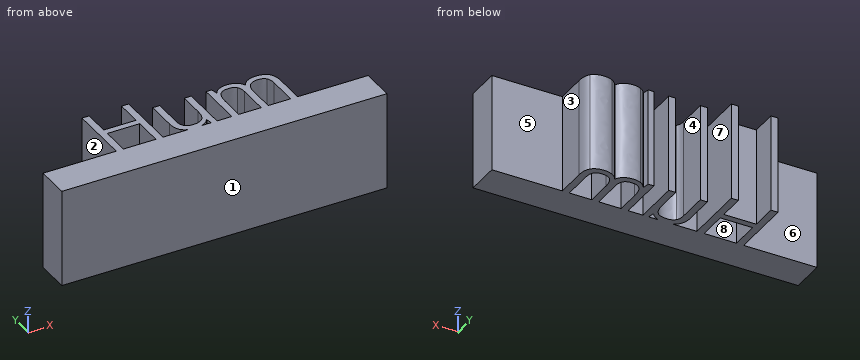
from build123d import *

# Parameters (mm, degrees)
F1_DEPTH = 15


with BuildPart() as f1:
    # F0 (on Top) → F1 (new body)
    with BuildSketch(Plane.XY):
        with BuildLine():
            Line((0, 5.1869419025), (0, 0))
            Line((0, 0), (50, 0))
            Line((50, 0), (50, 5.1869419025))
            Line((50, 5.1869419025), (39.1645775294, 5.1869419025))
            Line((39.1645775294, 5.1869419025), (38.091016748, 5.1869419025))
            Line((38.091016748, 5.1869419025), (34.6382131539, 5.1869419025))
            Line((34.6382131539, 5.1869419025), (33.5625798614, 5.1869419025))
            Line((33.5625798614, 5.1869419025), (30.1180663119, 5.1869419025))
            Line((30.1180663119, 5.1869419025), (29.0424330194, 5.1869419025))
            Line((29.0424330194, 5.1869419025), (26.7626707424, 5.1869419025))
            Line((26.7626707424, 5.1869419025), (25.8756359655, 5.1869419025))
            Line((25.8756359655, 5.1869419025), (24.3593894687, 5.1869419025))
            add(Edge.make_bspline(
                [(24.3593894687, 5.1869419025), (23.9221630132, 5.0563736994), (23.4072751728, 5.0563736994)],
                knots=[0.3156013684, 0.3156013684, 0.3156013684, 1, 1, 1], degree=2))
            add(Edge.make_bspline(
                [(23.4072751728, 5.0563736994), (22.8106948217, 5.0563736994), (22.3523760863, 5.1869419025)],
                knots=[0, 0, 0, 0.4605661865, 0.4605661865, 0.4605661865], degree=2))
            Line((22.3523760863, 5.1869419025), (18.4664085652, 5.1869419025))
            Line((18.4664085652, 5.1869419025), (17.3659051387, 5.1869419025))
            Line((17.3659051387, 5.1869419025), (12.3773707744, 5.1869419025))
            Line((12.3773707744, 5.1869419025), (11.2768673479, 5.1869419025))
            Line((11.2768673479, 5.1869419025), (0, 5.1869419025))
        make_face()
        Polygon((11.2768673479, 14.6562453968), (11.2768673479, 5.1869419025), (12.3773707744, 5.1869419025), (12.3773707744, 9.6428408985), (17.3659051387, 9.6428408985), (17.3659051387, 5.1869419025), (18.4664085652, 5.1869419025), (18.4664085652, 14.6562453968), (17.3659051387, 14.6562453968), (17.3659051387, 10.6272837), (12.3773707744, 10.6272837), (12.3773707744, 14.6562453968), align=None)
        with BuildLine():
            Line((38.091016748, 5.1869419025), (39.1645775294, 5.1869419025))
            Line((39.1645775294, 5.1869419025), (39.1645775294, 9.816931836))
            add(Edge.make_bspline(
                [(38.5656218039, 11.7972162503), (39.1645775294, 11.1785716688), (39.1645775294, 9.816931836)],
                knots=[0, 0, 0, 1, 1, 1], degree=2))
            add(Edge.make_bspline(
                [(36.7625370938, 12.4158608318), (37.9666660783, 12.4158608318), (38.5656218039, 11.7972162503)],
                knots=[0, 0, 0, 1, 1, 1], degree=2))
            add(Edge.make_bspline(
                [(35.3894984497, 12.0915128351), (35.991562942, 12.4158608318), (36.7625370938, 12.4158608318)],
                knots=[0, 0, 0, 1, 1, 1], degree=2))
            add(Edge.make_bspline(
                [(34.4703397499, 11.2096593362), (34.7874339575, 11.7671648385), (35.3894984497, 12.0915128351)],
                knots=[0, 0, 0, 1, 1, 1], degree=2))
            Line((34.4703397499, 11.2096593362), (34.4185269708, 11.2096593362))
            add(Edge.make_bspline(
                [(32.2423902519, 12.4158608318), (33.9066167141, 12.4158608318), (34.4185269708, 11.2096593362)],
                knots=[0, 0, 0, 1, 1, 1], degree=2))
            add(Edge.make_bspline(
                [(31.001992322, 12.1236367581), (31.5563890576, 12.4158608318), (32.2423902519, 12.4158608318)],
                knots=[0, 0, 0, 1, 1, 1], degree=2))
            add(Edge.make_bspline(
                [(30.1429364458, 11.3132848942), (30.4475955865, 11.8314126845), (31.001992322, 12.1236367581)],
                knots=[0, 0, 0, 1, 1, 1], degree=2))
            Line((30.1429364458, 11.3132848942), (30.0911236668, 11.3132848942))
            Line((30.0911236668, 11.3132848942), (29.9170327293, 12.2852926287))
            Line((29.9170327293, 12.2852926287), (29.0424330194, 12.2852926287))
            Line((29.0424330194, 12.2852926287), (29.0424330194, 5.1869419025))
            Line((29.0424330194, 5.1869419025), (30.1180663119, 5.1869419025))
            Line((30.1180663119, 5.1869419025), (30.1180663119, 8.9112444587))
            add(Edge.make_bspline(
                [(30.5874900899, 10.8967101509), (30.1180663119, 10.2915368919), (30.1180663119, 8.9112444587)],
                knots=[0, 0, 0, 1, 1, 1], degree=2))
            add(Edge.make_bspline(
                [(32.0662268032, 11.5018834099), (31.0569138678, 11.5018834099), (30.5874900899, 10.8967101509)],
                knots=[0, 0, 0, 1, 1, 1], degree=2))
            add(Edge.make_bspline(
                [(33.1998904082, 11.0780548775), (32.837200955, 11.5018834099), (32.0662268032, 11.5018834099)],
                knots=[0, 0, 0, 1, 1, 1], degree=2))
            add(Edge.make_bspline(
                [(33.5625798614, 9.8044967691), (33.5625798614, 10.654226345), (33.1998904082, 11.0780548775)],
                knots=[0, 0, 0, 1, 1, 1], degree=2))
            Line((33.5625798614, 9.8044967691), (33.5625798614, 5.1869419025))
            Line((33.5625798614, 5.1869419025), (34.6382131539, 5.1869419025))
            Line((34.6382131539, 5.1869419025), (34.6382131539, 9.1516557534))
            add(Edge.make_bspline(
                [(35.1179994877, 10.9257253071), (34.6382131539, 10.3495672044), (34.6382131539, 9.1516557534)],
                knots=[0, 0, 0, 1, 1, 1], degree=2))
            add(Edge.make_bspline(
                [(36.6008812233, 11.5018834099), (35.5977858214, 11.5018834099), (35.1179994877, 10.9257253071)],
                knots=[0, 0, 0, 1, 1, 1], degree=2))
            add(Edge.make_bspline(
                [(37.7283272948, 11.0780548775), (37.3656378417, 11.5018834099), (36.6008812233, 11.5018834099)],
                knots=[0, 0, 0, 1, 1, 1], degree=2))
            add(Edge.make_bspline(
                [(38.091016748, 9.8044967691), (38.091016748, 10.654226345), (37.7283272948, 11.0780548775)],
                knots=[0, 0, 0, 1, 1, 1], degree=2))
            Line((38.091016748, 9.8044967691), (38.091016748, 5.1869419025))
        make_face()
        with BuildLine():
            add(Edge.make_bspline(
                [(22.3523760863, 5.1869419025), (21.8155745788, 5.3398686822), (21.4684409818, 5.6719095142)],
                knots=[0.4605661865, 0.4605661865, 0.4605661865, 1, 1, 1], degree=2))
            Line((22.3523760863, 5.1869419025), (24.3593894687, 5.1869419025))
            add(Edge.make_bspline(
                [(24.7461173828, 5.3351264505), (24.5610106604, 5.2471517008), (24.3593894687, 5.1869419025)],
                knots=[0, 0, 0, 0.3156013684, 0.3156013684, 0.3156013684], degree=2))
            add(Edge.make_bspline(
                [(25.6621673159, 6.1382245254), (25.3326380413, 5.6138792017), (24.7461173828, 5.3351264505)],
                knots=[0, 0, 0, 1, 1, 1], degree=2))
            Line((25.6621673159, 6.1382245254), (25.7201976284, 6.1382245254))
            Line((25.7201976284, 6.1382245254), (25.8756359655, 5.1869419025))
            Line((25.8756359655, 5.1869419025), (26.7626707424, 5.1869419025))
            Line((26.7626707424, 5.1869419025), (26.7626707424, 12.2852926287))
            Line((26.7626707424, 12.2852926287), (25.6870374498, 12.2852926287))
            Line((25.6870374498, 12.2852926287), (25.6870374498, 8.554772539))
            add(Edge.make_bspline(
                [(25.1730546819, 6.5661980801), (25.6870374498, 7.1744801058), (25.6870374498, 8.554772539)],
                knots=[0, 0, 0, 1, 1, 1], degree=2))
            add(Edge.make_bspline(
                [(23.5440609094, 5.9579160544), (24.659071914, 5.9579160544), (25.1730546819, 6.5661980801)],
                knots=[0, 0, 0, 1, 1, 1], degree=2))
            add(Edge.make_bspline(
                [(22.307808002, 6.3848533535), (22.7026213781, 5.9579160544), (23.5440609094, 5.9579160544)],
                knots=[0, 0, 0, 1, 1, 1], degree=2))
            add(Edge.make_bspline(
                [(21.9129946258, 7.6801728291), (21.9129946258, 6.8117906527), (22.307808002, 6.3848533535)],
                knots=[0, 0, 0, 1, 1, 1], degree=2))
            Line((21.9129946258, 7.6801728291), (21.9129946258, 12.2852926287))
            Line((21.9129946258, 12.2852926287), (20.8249262663, 12.2852926287))
            Line((20.8249262663, 12.2852926287), (20.8249262663, 7.6407951171))
            add(Edge.make_bspline(
                [(21.4684409818, 5.6719095142), (20.8249262663, 6.287445329), (20.8249262663, 7.6407951171)],
                knots=[0, 0, 0, 1, 1, 1], degree=2))
        make_face()
        with BuildLine():
            Line((24.3593894687, 5.1869419025), (22.3523760863, 5.1869419025))
            add(Edge.make_bspline(
                [(23.4072751728, 5.0563736994), (22.8106948217, 5.0563736994), (22.3523760863, 5.1869419025)],
                knots=[0, 0, 0, 0.4605661865, 0.4605661865, 0.4605661865], degree=2))
            add(Edge.make_bspline(
                [(24.3593894687, 5.1869419025), (23.9221630132, 5.0563736994), (23.4072751728, 5.0563736994)],
                knots=[0.3156013684, 0.3156013684, 0.3156013684, 1, 1, 1], degree=2))
        make_face()
    extrude(amount=F1_DEPTH)


solid = f1.part
The listing builds one solid part. Answer for the finished solid, in the listing's coordinates (mm). Face numbers are marked on the shaded views. A direction names the side the tool comes from. Coordinates: 2 decimals unless noted, no trailing zeros. Loops run counter-clockwise (first coordinate to the right, second up) from the corner with the lowest first, then second, coordinate; pieces in that order, holes last. Notation, with made-up numbers: (54.25, 74) -> (107.25, 74) arc R16 ccw to (107.25, 95) -> close; hole circle Ø3 at (37.25, 71.5). An arc over 180 degrees is marked (long way). Write item = value, one per line. Start each with the question number.
1) A cutting plane is placed at A-A (y = 13.75). Give the vertices of the cut face in (x, z), then the cut area to 3 significant figures.
2) The mould has two halves that part along X. Classify the marked faces 1, 2, 3 and 4: released by +X, released by -X, zero draft, split by the parting line, or undercut.
3) Given pin 1 Ø3.5 at (y, z) = (7, 6.5) entering from -X; pin 2 Ø4 at (y, z) = (9.5, 10.5) entering from +X; pin 3 Ø0.9 at (x, z) = (26.5, 9.5) entering from +Y, each flat-ended and moving along its own axis, determine where each tip first touches the part or whether it passes through.
4) A cutting plane is placed at B-B (x = 15). Give the vertices of the cut face in (y, z).
5) Straight lines are drawn through the part: line 1 (X direction, y = 12.5, z = 11); line 2 (Y direction, x = 8, z = 5.5). For each, find the intervals that lie inside material, in ascending order. Write a range as from..to.
6) A cutting plane is placed at D-D (x = 44). Give the vertices of the cut face in (y, z).
7) A tool of negligible diameter and unlimited length cuts with its end or side. For the marked faces 5, 6, 7 and 8, from which of +Z, -Z, +X, -X, +Y, -Y can it reach the whole face along a straight path? Write none if from no direction.
8) A cutting plane is placed at C-C (z = 2.5). Count the separate pieces of the cut face and the enclosed holes in it, then the cut area to 3 significant figures.
Responses:
q1.outline = (11.28, 0) -> (12.38, 0) -> (12.38, 15) -> (11.28, 15) -> close; (17.37, 0) -> (18.47, 0) -> (18.47, 15) -> (17.37, 15) -> close
q1.area = 33.0 mm²
q2.face_1 = zero draft
q2.face_2 = released by -X
q2.face_3 = released by +X
q2.face_4 = undercut
q3.pin_1 = 11.28
q3.pin_2 = 39.16
q3.pin_3 = 12.29
q4.outline = (0, 0) -> (5.19, 0) -> (5.19, 15) -> (0, 15) -> close; (9.64, 0) -> (10.63, 0) -> (10.63, 15) -> (9.64, 15) -> close
q5.line_1 = 11.28..12.38, 17.37..18.47
q5.line_2 = 0..5.19
q6.outline = (0, 0) -> (5.19, 0) -> (5.19, 15) -> (0, 15) -> close
q7.face_5 = +Z, -Z, +X, +Y
q7.face_6 = +Z, -Z, -X, +Y
q7.face_7 = +Z, -Z, +Y
q7.face_8 = +Z, -Z
q8.separate_pieces = 1
q8.enclosed_holes = 4
q8.area = 332 mm²
